Build history of the part. All positions in model axes, mm. A direction names the side the tool comes from. Round coordinates to 2 decimals unless told otherwise and drop trailing zeros. Write each loop counter-clockwise with the first axis right and the second up, starting at its lowest first coordinate (ties: lowest second). Pieces come first, ordered by that corner, then holes. Notation, with made-up numbers: M 35,57.5 L 53,57.5 A16 cw 53,75.5 Z; hole C -2,59 d3. An arc over 180 degrees is marked long. Write item = value, one per line.
from build123d import *

# Parameters (mm, degrees)
F0_W     = 55
F0_H     = 12.2
F0_R     = 2.374951393
F0_R_2   = 2.1771962512
F1_DEPTH = 10
F2_W     = 20
F2_H     = 10
F3_DEPTH = 24
F4_R     = 2


with BuildPart() as f1:
    # F0 (on Front) → F1 (new body)
    with BuildSketch(Plane.XZ):
        Rectangle(F0_W, F0_H)
        with Locations((-21, 0)):
            Circle(F0_R, mode=Mode.SUBTRACT)
        with Locations((21, 0)):
            Circle(F0_R_2, mode=Mode.SUBTRACT)
    extrude(amount=F1_DEPTH)

    # F2 (on face) → F3 (join)
    with BuildSketch(Plane.XY.offset(6.1)):
        with Locations((0, -5)):
            Rectangle(F2_W, F2_H)
    extrude(amount=F3_DEPTH)

    # F4
    f4_edges = [f1.edges().sort_by_distance(p)[0] for p in [
        (10, -5, 6.1),
        (27.5, -5, 6.1),
        (27.5, -5, -6.1),
        (-10, -5, 6.1),
        (-27.5, -5, 6.1),
        (-27.5, -5, -6.1),
    ]]
    fillet(f4_edges, radius=F4_R)


solid = f1.part
1. Tool access for faces 5 (the face through (-10, -5, 19)), 6 (the face through (19, -5, 6.1)), 7 (the face through (0, -5, -6.1)): list every direction of +Z, -Z, +X, -X, +Y, -Y with a clear straight run to the whole face (end or side of a thin tool).
Responses:
face_5 = +Z, -X, +Y, -Y
face_6 = +Z, +X, +Y, -Y
face_7 = -Z, +X, -X, +Y, -Y
2. Band-saw the part on D-D (x = -21). List the corners of the cut face in (y, z).
Responses:
outline = M -10,-6.1 L 0,-6.1 L 0,-2.37 L -10,-2.37 Z; M -10,2.37 L 0,2.37 L 0,6.1 L -10,6.1 Z
3. Band-saw the part on A-A (x = 21). List the corners of the cut face in (y, z), plus the area to 3 significant figures.
Responses:
outline = M -10,-6.1 L 0,-6.1 L 0,-2.18 L -10,-2.18 Z; M -10,2.18 L 0,2.18 L 0,6.1 L -10,6.1 Z
area = 78.5 mm²
4. Mould opens along Z. For faces 1 (the face through (-27.5, -5, 0)), 2 (the face through (19.27, -4.93, -1.32)), 3 (the face through (-19, -5, 6.1)), 4 (the face through (-18.735, -4.93, 0.713)) say: pulls with the +Z half, pulls with the -Z half, needs draft (parallel to the pull), parting line crosses it, or undercut.
Responses:
face_1 = needs draft
face_2 = undercut
face_3 = pulls with the +Z half
face_4 = undercut
5. Flat gauge pins, fed straight in: pin 1 (6 mm diameter, centred on x = 0, z = 11.5, fed in from +Y); pin 2 (3 mm diameter, centred on y = -3.5, z = 17.5, fed in from +X); pin 3 (3 mm diameter, centred on y = -4.5, z = 23, fed in from -X). Where does each tip first touch, or does it go through?
Responses:
pin_1 = 0
pin_2 = 10
pin_3 = -10
6. Band-saw the part on B-B (y = -4). List the corners of the cut face in (x, z), plus the area to 3 significant figures.
Responses:
outline = M -27.5,-4.1 A2 ccw -25.5,-6.1 L 25.5,-6.1 A2 ccw 27.5,-4.1 L 27.5,4.1 A2 ccw 25.5,6.1 L 12,6.1 A2 cw 10,8.1 L 10,30.1 L -10,30.1 L -10,8.1 A2 cw -12,6.1 L -25.5,6.1 A2 ccw -27.5,4.1 Z; hole C -21,0 d4.75; hole C 21,0 d4.35
area = 1,120 mm²
7. Probe probe 1 along X at (y, z) = (-3.5, 1); probe 2 along X at (y, z) = (-5.75, 1.5); probe 3 along Z at (x, y) = (25.5, -5). List the from-to ranges inside material, lowest first.
Responses:
probe_1 = -27.5 to -23.15, -18.85 to 19.07, 22.93 to 27.5
probe_2 = -27.5 to -22.84, -19.16 to 19.42, 22.58 to 27.5
probe_3 = -6.1 to 6.1
8. Band-saw the part on C-C (z = 0). List the corners of the cut face in (x, y), plus the area to 3 significant figures.
Responses:
outline = M -27.5,-10 L -23.37,-10 L -23.37,0 L -27.5,0 Z; M -18.63,-10 L 18.82,-10 L 18.82,0 L -18.63,0 Z; M 23.18,-10 L 27.5,-10 L 27.5,0 L 23.18,0 Z
area = 459 mm²
